Verification items for the finished model (mm, model axes). A direction names the side the tool comes from. Give positions to 0.01 mm unless a question says otherwise; leave off trailing zeros. Write each loop counter-clockwise with the first axis right and the second up, starting at its lowest first coordinate (ties: lowest second). Pieces come first, ordered by that corner, then holes. Notation, with made-up numbers: (52, 62.25) - (106, 62.25) arc R20 cw to (106, 78.25) - close; hole circle Ø11 at (30, 1.25). An arc over 180 degrees is marked (long way). Answer as a JSON object with one key per item and string values. Group by question number.
Item 1: Sectioned sample at B-B, the plane x = -91.5. Record the boundary of the cut face in (y, z), and give its area (3 significant figures).
Item 2: Sectioned sample at C-C, the plane z = -12. Record the boundary of the cut face in (x, y), and give its area (3 significant figures).
Item 3: Scan lines: line 1 along Z through (x, y) = (-21, 28); line 2 along Y through (x, z) = (-77.5, -25.95); line 3 along Y through (x, z) = (-127.5, 1.2). Record each from-to range of solid material in increasing order. Write a range as [from, to].
Item 4: Sectioned sample at A-A, the plane x = -172. Record the boundary of the cut face in (y, z), and give its area (3 significant figures).
Item 5: Draft check along Y on faces 1 (the face through (-175.37, 5.53, 1.01)), 2 (the face through (-237, 36, -13)), 3 (the face through (196.99, -12.03, 0.99)), 4 (the face through (162.403, 8.375, 0.986)). Enter one of: +Y half, -Y half, draft (parallel to the pull), parting line (faces both ways), or undercut.
Item 6: Tool access check on faces 5 (the face through (-4, 35.335, -13)), 6 (the face through (189.597, 7.865, 0.986)), 7 (the face through (235, 36, -13)), 8 (the face through (142.85, -11.87, 0.99)), 9 (the face through (-4, 37.335, -13)). Record the directions out of +Z, -Z, +X, -X, +Y, -Y that give a thin tool (end or side, any length) a straight path to the whole face; none if there is none.
Item 7: Go/stop test with flat-tipped pins: pin 1 (1.6 mm diameter, centred on y = 9, z = 1, fed in from -X); pin 2 (2.5 mm diameter, centred on x = 72.5, y = 25.33, fed in from +Z); pin 3 (6 mm diameter, centred on x = -163, y = 14.5, fed in from -Z); pin 4 (9 mm diameter, centred on x = 193.1, z = -20.23, fed in from +Y). Record where each tip stops, or that it passes through.
```python
from build123d import *

# Parameters (mm, degrees)
BOSS_EXTRUDE1_DEPTH        = 2
SKETCH2_W                  = 400
SKETCH2_H                  = 2
BOSS_EXTRUDE2_DEPTH        = 37
CUT_EXTRUDE7_REACH         = 217.461
SKETCH32_W                 = 50
SKETCH32_H                 = 10
SKETCH35_W                 = 37
SKETCH35_H                 = 40
BOSS_EXTRUDE7_DEPTH        = 2
SKETCHED_START             = -237
SKETCHED_BEND1_DEPTH       = 472
SKETCHED_BEND1_2_DEPTH     = 472
SKETCHED_START_2           = -200
SKETCHED_BEND1_3_OUTLINE_W = 10
SKETCHED_BEND1_3_OUTLINE_H = 2
SKETCHED_BEND1_3_DEPTH     = 350
SKETCH24_W                 = 300
SKETCH24_H                 = 12
CUT_EXTRUDE4_DEPTH         = 1
CUT_EXTRUDE5_REACH         = 243.721
SKETCH25_R                 = 4.25
SKETCH30_W                 = 300
SKETCH30_H                 = 12
BOSS_EXTRUDE6_DEPTH        = 1
M3_5_TAPPED_HOLE1_D        = 2.9
LPATTERN1_COUNT            = 12
LPATTERN1_PITCH            = 25
SKETCH31_R                 = 2.25
CUT_EXTRUDE6_DEPTH         = 242.485502568
CUT_EXTRUDE8_REACH         = 246.229
SKETCH38_R                 = 2.75


# Read off the part's stored shape, not the designer's step: Sketched Bend1
with BuildPart() as part:
    # Sketch1 → Boss-Extrude1 (new body)
    with BuildSketch(Plane.XY):
        with BuildLine():
            Line((-190, -14.879809267), (-150, -14.879809267))
            ThreePointArc((-150, -14.879809267), (-142.928932188, -11.950877079), (-140, -4.879809267))
            Line((-140, -4.879809267), (-140, 18.120190733))
            Line((-140, 18.120190733), (140, 18.120190733))
            Line((140, 18.120190733), (140, -4.879809267))
            ThreePointArc((140, -4.879809267), (142.928932188, -11.950877079), (150, -14.879809267))
            Line((150, -14.879809267), (190, -14.879809267))
            ThreePointArc((190, -14.879809267), (197.071067812, -11.950877079), (200, -4.879809267))
            Line((200, -4.879809267), (200, 43.120190733))
            Line((200, 43.120190733), (-200, 43.120190733))
            Line((-200, 43.120190733), (-200, -4.879809267))
            ThreePointArc((-200, -4.879809267), (-197.071067812, -11.950877079), (-190, -14.879809267))
        make_face()
        with BuildLine():
            Line((178, 19.720190733), (174, 19.720190733))
            ThreePointArc((174, 19.720190733), (162.4, 8.120190733), (174, -3.479809267))
            Line((174, -3.479809267), (178, -3.479809267))
            ThreePointArc((178, -3.479809267), (189.6, 8.120190733), (178, 19.720190733))
        make_face(mode=Mode.SUBTRACT)
        with BuildLine():
            Line((158.5, -5.779809267), (162.5, -5.779809267))
            ThreePointArc((162.5, -5.779809267), (164.1, -7.379809267), (162.5, -8.979809267))
            Line((162.5, -8.979809267), (158.5, -8.979809267))
            ThreePointArc((158.5, -8.979809267), (156.9, -7.379809267), (158.5, -5.779809267))
        make_face(mode=Mode.SUBTRACT)
        with BuildLine():
            Line((193.5, -5.779809267), (189.5, -5.779809267))
            ThreePointArc((189.5, -5.779809267), (187.9, -7.379809267), (189.5, -8.979809267))
            Line((189.5, -8.979809267), (193.5, -8.979809267))
            ThreePointArc((193.5, -8.979809267), (195.1, -7.379809267), (193.5, -5.779809267))
        make_face(mode=Mode.SUBTRACT)
        with BuildLine():
            Line((193.5, 25.220190733), (189.5, 25.220190733))
            ThreePointArc((189.5, 25.220190733), (187.9, 23.620190733), (189.5, 22.020190733))
            Line((189.5, 22.020190733), (193.5, 22.020190733))
            ThreePointArc((193.5, 22.020190733), (195.1, 23.620190733), (193.5, 25.220190733))
        make_face(mode=Mode.SUBTRACT)
        with BuildLine():
            Line((158.5, 25.220190733), (162.5, 25.220190733))
            ThreePointArc((162.5, 25.220190733), (164.1, 23.620190733), (162.5, 22.020190733))
            Line((162.5, 22.020190733), (158.5, 22.020190733))
            ThreePointArc((158.5, 22.020190733), (156.9, 23.620190733), (158.5, 25.220190733))
        make_face(mode=Mode.SUBTRACT)
    extrude(amount=BOSS_EXTRUDE1_DEPTH)

    # Sketch2 → Boss-Extrude2 (add)
    with BuildSketch(Plane(origin=(0, 43.120190733, 40.120190733), x_dir=(-1, 0, 0), z_dir=(0, -1, 0))):
        with Locations((0, 39.120190733)):
            Rectangle(SKETCH2_W, SKETCH2_H)
    extrude(amount=-BOSS_EXTRUDE2_DEPTH)

    # Sketch32 → Cut-Extrude7 (cut, up to next)
    with BuildSketch(Plane.XY.offset(2), mode=Mode.PRIVATE) as cut_extrude7_sk1:
        with Locations((175, 75.120190733)):
            Rectangle(SKETCH32_W, SKETCH32_H)
    cut_extrude7_tool1 = extrude(cut_extrude7_sk1.sketch, amount=-CUT_EXTRUDE7_REACH, mode=Mode.PRIVATE) & part.part
    add(cut_extrude7_tool1.solids().sort_by_distance((175, 75.120191, 2))[0], mode=Mode.SUBTRACT)

    # Sketch35 → Boss-Extrude7 (add)
    with BuildSketch(Plane(origin=(0, 0, 0), x_dir=(-1, 0, 0), z_dir=(0, 0, -1))):
        with Locations((-216.5, 50.120190733)):
            Rectangle(SKETCH35_W, SKETCH35_H)
        with Locations((218.5, 50.120190733)):
            Rectangle(SKETCH35_W, SKETCH35_H)
    extrude(amount=-BOSS_EXTRUDE7_DEPTH)

    # Sketched Bend1 outline → Sketched Bend1 (cut)
    with BuildSketch(Plane.YZ.offset(SKETCHED_START)):
        with BuildLine():
            ThreePointArc((35.33479257, 2), (36.749006132, 1.414213562), (37.33479257, 0))
            Line((37.33479257, 0), (80.120190733, 0))
            Line((80.120190733, 0), (80.120190733, 2))
            Line((80.120190733, 2), (35.33479257, 2))
        make_face()
    extrude(amount=SKETCHED_BEND1_DEPTH, mode=Mode.SUBTRACT)

    # Sketched Bend1 2 outline → Sketched Bend1 2 (add)
    with BuildSketch(Plane.YZ.offset(SKETCHED_START)):
        with BuildLine():
            ThreePointArc((35.33479257, -27.429203673), (36.749006132, -26.843417235), (37.33479257, -25.429203673))
            Line((37.33479257, -25.429203673), (37.33479257, 0))
            Line((37.33479257, 0), (35.33479257, 0))
            Line((35.33479257, 0), (35.33479257, -25.429203673))
            Line((35.33479257, -25.429203673), (29.120190733, -25.429203673))
            Line((29.120190733, -25.429203673), (29.120190733, -27.429203673))
            Line((29.120190733, -27.429203673), (35.33479257, -27.429203673))
        make_face()
    extrude(amount=SKETCHED_BEND1_2_DEPTH)

    # Sketched Bend1 3 outline → Sketched Bend1 3 (add)
    with BuildSketch(Plane.YZ.offset(SKETCHED_START_2)):
        with Locations((24.120190733, -26.429203673)):
            Rectangle(SKETCHED_BEND1_3_OUTLINE_W, SKETCHED_BEND1_3_OUTLINE_H)
    extrude(amount=SKETCHED_BEND1_3_DEPTH)

    # Sketch24 → Cut-Extrude4 (cut)
    with BuildSketch(Plane.XY.offset(2)):
        with Locations((0, 27.33479257)):
            Rectangle(SKETCH24_W, SKETCH24_H)
    extrude(amount=-CUT_EXTRUDE4_DEPTH, mode=Mode.SUBTRACT)

    # Sketch25 → Cut-Extrude5 (cut, up to next)
    with BuildSketch(Plane.XY.offset(2), mode=Mode.PRIVATE) as cut_extrude5_sk1:
        with Locations((-172, 8.120190733)):
            Circle(SKETCH25_R)
    cut_extrude5_tool1 = extrude(cut_extrude5_sk1.sketch, amount=-CUT_EXTRUDE5_REACH, mode=Mode.PRIVATE) & part.part
    add(cut_extrude5_tool1.solids().sort_by_distance((-172, 8.120191, 2))[0], mode=Mode.SUBTRACT)

    # Sketch30 → Boss-Extrude6 (add)
    with BuildSketch(Plane.XY.offset(1)):
        with Locations((0, 27.33479257)):
            Rectangle(SKETCH30_W, SKETCH30_H)
    extrude(amount=BOSS_EXTRUDE6_DEPTH)

    # M3.5 Tapped Hole1 (through all)
    with Locations(Plane(origin=(-127.5, 25.33479257, 2), x_dir=(1, 0, 0), z_dir=(0, 0, 1))):
        with Locations((0, 0)):
            m3_5_tapped_hole1 = Hole(M3_5_TAPPED_HOLE1_D / 2)

    # LPattern1: M3.5 Tapped Hole1 ×12
    with Locations(*[(i * LPATTERN1_PITCH, 0, 0) for i in range(1, LPATTERN1_COUNT)]):
        add(m3_5_tapped_hole1, mode=Mode.SUBTRACT)

    # Sketch31 → Cut-Extrude6 (cut, through all)
    with BuildSketch(Plane(origin=(0, 0, 0), x_dir=(-1, 0, 0), z_dir=(0, 0, -1))):
        with Locations((190.5, 8.120190733)):
            Circle(SKETCH31_R)
        with Locations((153.5, 8.120190733)):
            Circle(SKETCH31_R)
    extrude(amount=-CUT_EXTRUDE6_DEPTH, mode=Mode.SUBTRACT)

    # Sketch38 → Cut-Extrude8 (cut, up to next)
    with BuildSketch(Plane(origin=(0, 37.33479257, 0), x_dir=(1, 0, 0), z_dir=(0, 1, 0)), mode=Mode.PRIVATE) as cut_extrude8_sk1:
        with Locations(Location((193.10140085, 5.229203673, 0), (0, 0, 270))):
            Circle(SKETCH38_R)
    cut_extrude8_tool1 = extrude(cut_extrude8_sk1.sketch, amount=-CUT_EXTRUDE8_REACH, mode=Mode.PRIVATE) & part.part
    # Sketch38 → Cut-Extrude8 (cut, up to next)
    with BuildSketch(Plane(origin=(0, 37.33479257, 0), x_dir=(1, 0, 0), z_dir=(0, 1, 0)), mode=Mode.PRIVATE) as cut_extrude8_sk2:
        with Locations(Location((193.10140085, 20.229203673, 0), (0, 0, 270))):
            Circle(SKETCH38_R)
    cut_extrude8_tool2 = extrude(cut_extrude8_sk2.sketch, amount=-CUT_EXTRUDE8_REACH, mode=Mode.PRIVATE) & part.part
    # Sketch38 → Cut-Extrude8 (cut, up to next)
    with BuildSketch(Plane(origin=(0, 37.33479257, 0), x_dir=(1, 0, 0), z_dir=(0, 1, 0)), mode=Mode.PRIVATE) as cut_extrude8_sk3:
        with Locations(Location((217.5, 20.229203673, 0), (0, 0, 270))):
            Circle(SKETCH38_R)
    cut_extrude8_tool3 = extrude(cut_extrude8_sk3.sketch, amount=-CUT_EXTRUDE8_REACH, mode=Mode.PRIVATE) & part.part
    # Sketch38 → Cut-Extrude8 (cut, up to next)
    with BuildSketch(Plane(origin=(0, 37.33479257, 0), x_dir=(1, 0, 0), z_dir=(0, 1, 0)), mode=Mode.PRIVATE) as cut_extrude8_sk4:
        with Locations(Location((217.5, 5.229203673, 0), (0, 0, 270))):
            Circle(SKETCH38_R)
    cut_extrude8_tool4 = extrude(cut_extrude8_sk4.sketch, amount=-CUT_EXTRUDE8_REACH, mode=Mode.PRIVATE) & part.part
    # Sketch38 → Cut-Extrude8 (cut, up to next)
    with BuildSketch(Plane(origin=(0, 37.33479257, 0), x_dir=(1, 0, 0), z_dir=(0, 1, 0)), mode=Mode.PRIVATE) as cut_extrude8_sk5:
        with Locations(Location((-219.5, 5.229203673, 0), (0, 0, 270))):
            Circle(SKETCH38_R)
    cut_extrude8_tool5 = extrude(cut_extrude8_sk5.sketch, amount=-CUT_EXTRUDE8_REACH, mode=Mode.PRIVATE) & part.part
    # Sketch38 → Cut-Extrude8 (cut, up to next)
    with BuildSketch(Plane(origin=(0, 37.33479257, 0), x_dir=(1, 0, 0), z_dir=(0, 1, 0)), mode=Mode.PRIVATE) as cut_extrude8_sk6:
        with Locations(Location((-219.5, 20.229203673, 0), (0, 0, 270))):
            Circle(SKETCH38_R)
    cut_extrude8_tool6 = extrude(cut_extrude8_sk6.sketch, amount=-CUT_EXTRUDE8_REACH, mode=Mode.PRIVATE) & part.part
    # Sketch38 → Cut-Extrude8 (cut, up to next)
    with BuildSketch(Plane(origin=(0, 37.33479257, 0), x_dir=(1, 0, 0), z_dir=(0, 1, 0)), mode=Mode.PRIVATE) as cut_extrude8_sk7:
        with Locations(Location((-195.10140085, 20.229203673, 0), (0, 0, 270))):
            Circle(SKETCH38_R)
    cut_extrude8_tool7 = extrude(cut_extrude8_sk7.sketch, amount=-CUT_EXTRUDE8_REACH, mode=Mode.PRIVATE) & part.part
    # Sketch38 → Cut-Extrude8 (cut, up to next)
    with BuildSketch(Plane(origin=(0, 37.33479257, 0), x_dir=(1, 0, 0), z_dir=(0, 1, 0)), mode=Mode.PRIVATE) as cut_extrude8_sk8:
        with Locations(Location((-195.10140085, 5.229203673, 0), (0, 0, 270))):
            Circle(SKETCH38_R)
    cut_extrude8_tool8 = extrude(cut_extrude8_sk8.sketch, amount=-CUT_EXTRUDE8_REACH, mode=Mode.PRIVATE) & part.part
    add(cut_extrude8_tool1.solids().sort_by_distance((193.101401, 37.334793, -5.229204))[0], mode=Mode.SUBTRACT)
    add(cut_extrude8_tool2.solids().sort_by_distance((193.101401, 37.334793, -20.229204))[0], mode=Mode.SUBTRACT)
    add(cut_extrude8_tool3.solids().sort_by_distance((217.5, 37.334793, -20.229204))[0], mode=Mode.SUBTRACT)
    add(cut_extrude8_tool4.solids().sort_by_distance((217.5, 37.334793, -5.229204))[0], mode=Mode.SUBTRACT)
    add(cut_extrude8_tool5.solids().sort_by_distance((-219.5, 37.334793, -5.229204))[0], mode=Mode.SUBTRACT)
    add(cut_extrude8_tool6.solids().sort_by_distance((-219.5, 37.334793, -20.229204))[0], mode=Mode.SUBTRACT)
    add(cut_extrude8_tool7.solids().sort_by_distance((-195.101401, 37.334793, -20.229204))[0], mode=Mode.SUBTRACT)
    add(cut_extrude8_tool8.solids().sort_by_distance((-195.101401, 37.334793, -5.229204))[0], mode=Mode.SUBTRACT)


solid = part.part
```
Geometry check:
{
 "1": {"outline": "(18.12, 0) - (35.33, 0) - (35.33, -25.43) - (19.12, -25.43) - (19.12, -27.43) - (35.33, -27.43) arc R2 ccw to (37.33, -25.43) - (37.33, 0) arc R2 ccw to (35.33, 2) - (18.12, 2) - close", "area": "124 mm^2"},
 "2": {"outline": "(-237, 35.33) - (235, 35.33) - (235, 37.33) - (-237, 37.33) - close", "area": "944 mm^2"},
 "3": {"line 1": "[-27.43, -25.43], [0, 2]", "line 2": "[19.12, 23.88], [26.78, 37.27]", "line 3": "[18.12, 23.88], [26.78, 36.93]"},
 "4": {"outline": "(-14.88, 0) - (3.87, 0) - (3.87, 2) - (-14.88, 2) - close; (12.37, 0) - (35.33, 0) - (35.33, -25.43) - (19.12, -25.43) - (19.12, -27.43) - (35.33, -27.43) arc R2 ccw to (37.33, -25.43) - (37.33, 0) arc R2 ccw to (35.33, 2) - (12.37, 2) - close", "area": "173 mm^2"},
 "5": {"face 1": "undercut", "face 2": "draft", "face 3": "-Y half", "face 4": "undercut"},
 "6": {"face 5": "+X, -X, -Y", "face 6": "+Z, -Z", "face 7": "+Z, -Z, +X, +Y, -Y", "face 8": "+Z, -Z, -Y", "face 9": "+Z, -Z, +X, -X, +Y"},
 "7": {"pin 1": "x = -200", "pin 2": "through", "pin 3": "z = 0", "pin 4": "y = 37.33"}
}
